The model under review builds one solid part; all positions refer to its coordinate system, in mm. A direction names the side the tool comes from. Give positions to 0.01 mm unless a question says otherwise; leave off trailing zeros. Write each loop counter-clockwise with the first axis right and the second up, starting at its lowest first coordinate (ties: lowest second). Pieces come first, ordered by that corner, then holes. Notation, with made-up numbers: (22, 15) - (53, 15) arc R17 ccw to (53, 33) - close; hole circle Ø10 at (-24, 20.25). An arc over 180 degrees is marked (long way). Write item = value, one per line.
```python
from build123d import *

# Parameters (mm, degrees)
ESQUISSE1_W          = 101
ESQUISSE1_H          = 113
BOSS_EXTRU_1_DEPTH   = 5
D_GAGEMENT_M42_D     = 4.5
M4_CLEARANCE_HOLE1_D = 4.5
CUT_EXTRUDE1_DEPTH   = 76.944058359


with BuildPart() as part:
    # Esquisse1 → Boss.-Extru.1 (new body)
    with BuildSketch(Plane.XY):
        Rectangle(ESQUISSE1_W, ESQUISSE1_H)
    extrude(amount=BOSS_EXTRU_1_DEPTH)

    # Dégagement M42 (through all)
    with Locations(Plane.XY.offset(5)):
        with Locations((-20.723129893, -30.91293976), (-20.723129893, 3.803464199), (-41.035821543, 3.803464199), (-41.035821543, -30.91293976), (-41.035821543, 35.983767161), (-20.723129893, 35.983767161)):
            Hole(D_GAGEMENT_M42_D / 2)

    # M4 Clearance Hole1 (through all)
    with Locations(Plane.XY.offset(5)):
        with Locations((44.8, 51.5), (12.8, 51.5), (12.8, -51.5), (44.8, -51.5)):
            Hole(M4_CLEARANCE_HOLE1_D / 2)

    # Sketch3 → Cut-Extrude1 (cut, through all)
    with BuildSketch(Plane.XY.offset(5)):
        with BuildLine():
            Line((45.008341295, 28.5), (45.008341295, -28.5))
            ThreePointArc((45.008341295, -28.5), (43.83676842, -31.328427125), (41.008341295, -32.5))
            Line((41.008341295, -32.5), (17.008341295, -32.5))
            ThreePointArc((17.008341295, -32.5), (14.17991417, -31.328427125), (13.008341295, -28.5))
            Line((13.008341295, -28.5), (13.008341295, 28.5))
            ThreePointArc((13.008341295, 28.5), (14.17991417, 31.328427125), (17.008341295, 32.5))
            Line((17.008341295, 32.5), (41.008341295, 32.5))
            ThreePointArc((41.008341295, 32.5), (43.83676842, 31.328427125), (45.008341295, 28.5))
        make_face()
    extrude(amount=-CUT_EXTRUDE1_DEPTH, mode=Mode.SUBTRACT)


solid = part.part
```
1. Draft analysis for pull direction Y (two halves, no side actions). For faces 3 (the cylindrical face through (46.46, -49.98, 2.47)), 4 (the flat face through (-1, -56.5, 2)), 5 (the flat face through (-12, 1, 5)), state which applies: +Y half, -Y half, draft (parallel to the pull), parting line (faces both ways), or undercut.
Findings below:
face_3 = undercut
face_4 = -Y half
face_5 = draft
2. Take a section at A-A on y = 11.5. Give the boundary of the cut face in (x, z), and give its area (3 significant figures).
Findings below:
outline = (-50.5, 0) - (13.01, 0) - (13.01, 5) - (-50.5, 5) - close; (45.01, 0) - (50.5, 0) - (50.5, 5) - (45.01, 5) - close
area = 345 mm²
3. Take a section at B-B on y = -51.5. Give the boundary of the cut face in (x, z).
Findings below:
outline = (-50.5, 0) - (10.55, 0) - (10.55, 5) - (-50.5, 5) - close; (15.05, 0) - (42.55, 0) - (42.55, 5) - (15.05, 5) - close; (47.05, 0) - (50.5, 0) - (50.5, 5) - (47.05, 5) - close
4. Take a section at D-D on z = 3.1. Count the separate pieces of the cut face and the enclosed holes in it, and give its area (3 significant figures).
Findings below:
separate_pieces = 1
enclosed_holes = 11
area = 9,190 mm²
5. Take a section at C-C on x = 30.5. Give the boundary of the cut face in (y, z), and give its area (3 significant figures).
Findings below:
outline = (-56.5, 0) - (-32.5, 0) - (-32.5, 5) - (-56.5, 5) - close; (32.5, 0) - (56.5, 0) - (56.5, 5) - (32.5, 5) - close
area = 240 mm²
6. For line 1 (X direction, y = -16, z = 3.65); line 2 (Y direction, x = 37, z = 0.35); line 3 (X direction, y = -52, z = 0.6), list the stretches that pass through material, from the lowest coordinate up. Write a range as from..to.
Findings below:
line_1 = -50.5..13.01, 45.01..50.5
line_2 = -56.5..-32.5, 32.5..56.5
line_3 = -50.5..10.61, 14.99..42.61, 46.99..50.5
7. Machinability: for faces 1 (the flat face through (-50.5, -1, 2)), 2 (the flat face through (29, -32.5, 3)), which of the approach directions +Z, -Z, +X, -X, +Y, -Y give a long, thin tool a straight path to every point of the face, cutting with its end or side? Answer none if there is none.
Findings below:
face_1 = +Z, -Z, -X, +Y, -Y
face_2 = +Z, -Z
